```python
from build123d import *

# Parameters (mm, degrees)
SKETCH_1_W          = 100.4
SKETCH_1_H          = 100.4
EXTRUDE_2_DEPTH     = 2
SKETCH_2_W          = 100.4
SKETCH_2_H          = 2
EXTRUDE_3_DEPTH     = 4
SKETCH_3_W          = 2
SKETCH_3_H          = 96.4
EXTRUDE_4_DEPTH     = 4
SKETCH_4_W          = 12
SKETCH_4_H          = 12
EXTRUDE_5_DEPTH     = 22.09
SKETCH_7_W          = 6
SKETCH_7_H          = 6
CUT_EXTRUDE_1_DEPTH = 22.09
SKETCH_8_W          = 6
SKETCH_8_H          = 6
EXTRUDE_6_DEPTH     = 2
SKETCH_10_W         = 100.4
SKETCH_10_H         = 100.4
EXTRUDE_7_DEPTH     = 1


with BuildPart() as part:
    # 草圖1 → 填料-伸長2 (new body)
    with BuildSketch(Plane.XY):
        with Locations((50.2, -50.2)):
            Rectangle(SKETCH_1_W, SKETCH_1_H)
    extrude(amount=EXTRUDE_2_DEPTH)

    # 草圖2 → 填料-伸長3 (add)
    with BuildSketch(Plane.XY.offset(2)):
        Polygon((100.4, -2), (100.4, 0), (0, 0), (0, -2), (1, -2), (55.6, -2), align=None)
        with Locations((50.2, -99.4)):
            Rectangle(SKETCH_2_W, SKETCH_2_H)
    extrude(amount=EXTRUDE_3_DEPTH)

    # 草圖3 → 填料-伸長4 (add)
    with BuildSketch(Plane.XY.offset(2)):
        with Locations((1, -50.2)):
            Rectangle(SKETCH_3_W, SKETCH_3_H)
        with Locations((99.4, -50.2)):
            Rectangle(SKETCH_3_W, SKETCH_3_H)
    extrude(amount=EXTRUDE_4_DEPTH)

    # 草圖4 → 填料-伸長5 (add)
    with BuildSketch(Plane.XY.offset(2)):
        with Locations((45.2, -62.1)):
            Rectangle(SKETCH_4_W, SKETCH_4_H)
    extrude(amount=EXTRUDE_5_DEPTH)

    # 草圖7 → 除料-伸長1 (cut)
    with BuildSketch(Plane.XY.offset(24.09)):
        with Locations((45.2, -62.1)):
            Rectangle(SKETCH_7_W, SKETCH_7_H)
    extrude(amount=-CUT_EXTRUDE_1_DEPTH, mode=Mode.SUBTRACT)

    # 草圖8 → 填料-伸長6 (add)
    with BuildSketch(Plane.XY.offset(2)):
        with Locations((45.2, -62.1)):
            Rectangle(SKETCH_8_W, SKETCH_8_H)
    extrude(amount=EXTRUDE_6_DEPTH)

    # 草圖10 → 填料-伸長7 (add)
    with BuildSketch(Plane(origin=(0, 0, 0), x_dir=(-1, 0, 0), z_dir=(0, 0, -1))):
        with Locations((-50.2, -50.2)):
            Rectangle(SKETCH_10_W, SKETCH_10_H)
    extrude(amount=EXTRUDE_7_DEPTH)


solid = part.part
```
The listing builds one solid part. Answer for the finished solid, in the listing's coordinates (mm). A direction names the side the tool comes from. Give positions to 0.01 mm unless a question says otherwise; leave off trailing zeros. Order: outer loops, then holes, each group sorted by start corner. A loop starts at its lowest first (then second) coordinate and runs counter-clockwise, first axis right, second up. Notation, with made-up numbers: (-21, 47.5) -> (-6, 47.5) arc R17 ccw to (-6, 69.5) -> close; hole circle Ø4 at (-38.75, -12.5). An arc over 180 degrees is marked (long way). Answer as a JSON object with one key per item and string values. Group by question number.
Item 1: The part is cut by section C-C on x = 11.5. Write down the section's boundary in (y, z).
Item 2: The part is cut by section B-B on z = 21. Write down the section's boundary in (x, y), and give its area (3 significant figures).
Item 3: Consider L1, parallel to Y at x = 14.5, z = 2.5; L2, parallel to X at y = -70, z = 4.75; L3, parallel to Z at x = 70, y = -44. Determine where each line is inside the solid, lowest interval first. Write a range as from..to.
Item 4: The part is cut by section A-A on y = -77. Write down the section's boundary in (x, z).
Item 5: Determine the mould class of faces 1 (the flat face through (100.4, -51, 3)), 2 (the flat face through (51, -100.4, 3)), 3 (the flat face through (45, -59.1, 14)) for opening direction X: pulls with the +X half, pulls with the -X half, needs draft (parallel to the pull), parting line crosses it, or undercut.
Item 6: A tool of negligible diameter and unlimited length cuts with its end or side. For faces 4 (the flat face through (45, -56.1, 13)), 5 (the flat face through (51, 0, 3)), from which of +Z, -Z, +X, -X, +Y, -Y can it reach the whole face along a straight path? Write none if from no direction.
Item 7: Flat-ended cylindrical pins translate along their axes: pin 1 (3.5 mm diameter, centred on y = -63, z = 16, fed in from +X); pin 2 (6 mm diameter, centred on x = 80, y = -67.5, fed in from +Z); pin 3 (1.5 mm diameter, centred on y = -73.5, z = 7.5, fed in from -X); pin 4 (1.8 mm diameter, centred on x = 46, y = -63, fed in from +Z). Find the tip coordinate at first contact, or state that the pin passes through.
Result set:
{
 "1": {"outline": "(-100.4, -1) -> (0, -1) -> (0, 6) -> (-2, 6) -> (-2, 2) -> (-98.4, 2) -> (-98.4, 6) -> (-100.4, 6) -> close"},
 "2": {"outline": "(39.2, -68.1) -> (51.2, -68.1) -> (51.2, -56.1) -> (39.2, -56.1) -> close; hole (42.2, -65.1) -> (48.2, -65.1) -> (48.2, -59.1) -> (42.2, -59.1) -> close", "area": "108 mm²"},
 "3": {"L1": "-100.4..-98.4, -2..0", "L2": "0..2, 98.4..100.4", "L3": "-1..2"},
 "4": {"outline": "(0, -1) -> (100.4, -1) -> (100.4, 6) -> (98.4, 6) -> (98.4, 2) -> (2, 2) -> (2, 6) -> (0, 6) -> close"},
 "5": {"face 1": "pulls with the +X half", "face 2": "needs draft", "face 3": "undercut"},
 "6": {"face 4": "+Z", "face 5": "+Z, -Z, +X, -X, +Y"},
 "7": {"pin 1": "x = 51.2", "pin 2": "z = 2", "pin 3": "through", "pin 4": "z = 4"}
}
